from build123d import *

# Parameters (mm, degrees)
SKETCH_3_W          = 15
SKETCH_3_H          = 131.91272758
EXTRUDE_2_DEPTH     = 6.95
SKETCH_4_W          = 60
SKETCH_4_H          = 15
EXTRUDE_3_DEPTH     = 6.95
SKETCH_5_R          = 4.8
CUT_EXTRUDE_5_DEPTH = 7.95


with BuildPart() as part:
    # 草图3 → 凸台-拉伸2 (new body)
    with BuildSketch(Plane.XY):
        with Locations((-3.781807483, 0)):
            Rectangle(SKETCH_3_W, SKETCH_3_H)
    extrude(amount=EXTRUDE_2_DEPTH)

    # 草图4 → 凸台-拉伸3 (add)
    with BuildSketch(Plane.XY):
        with Locations((33.718192517, 58.45636379)):
            Rectangle(SKETCH_4_W, SKETCH_4_H)
    extrude(amount=EXTRUDE_3_DEPTH)

    # 草图5 → 切除-拉伸5 (cut, through all)
    with BuildSketch(Plane.XY):
        with Locations((-3.781807483, -54.073012812)):
            Circle(SKETCH_5_R)
    extrude(amount=CUT_EXTRUDE_5_DEPTH, mode=Mode.SUBTRACT)


solid = part.part
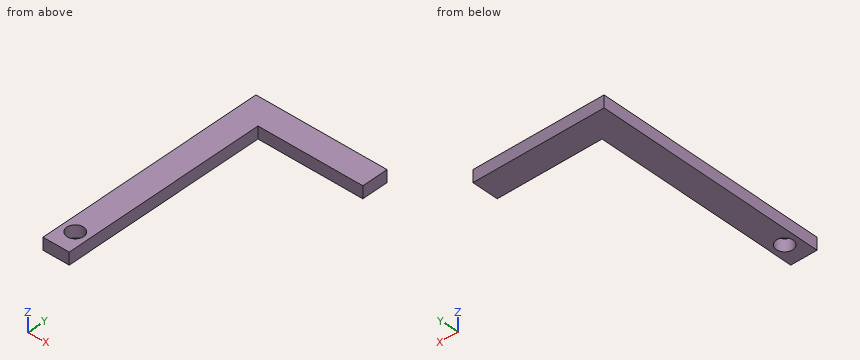
Design review of the part built by this model. Coordinates are the model's own, in mm. Give positions to 0.01 mm unless a question says otherwise; leave off trailing zeros. Loops run counter-clockwise (first coordinate to the right, second up) from the corner with the lowest first, then second, coordinate; pieces in that order, holes last. Notation, with made-up numbers: (6, 65) -> (17, 65) arc R21 ccw to (17, 98) -> close; hole circle Ø10 at (39, -28). An arc over 180 degrees is marked (long way). One line per question, with ' | ' between items. Start each with the question number.
(1) We need section C-C (z = 3.25). State the section outline as (x, y) points, and give its area (3 significant figures).
(2) For line 1 (X direction, y = 14, z = 4.25); line 2 (Y direction, x = 11.5, z = 3.25), list the stretches that pass through material, from the lowest coordinate up.
(3) We need section A-A (y = -51). State the section outline as (x, z) points.
(4) We need section B-B (x = -6). State the section outline as (y, z) points, and give its area (3 significant figures).
(5) We need section D-D (y = 26). State the section outline as (x, z) points.
(6) Insertion check: P1, Ø8.5, axis at x = -3.78, y = -54.07, coming from the +Z side; P2, Ø12, axis at x = 24, y = 46.5, coming from the -Z side; P3, Ø2, axis at y = -4, z = 4.5, coming from the +X side. Each pin has a flat end and moves straight along its axis. Give the tip position at first contact, or say it passes through.
The answers:
1) outline: (-11.28, -65.96) -> (3.72, -65.96) -> (3.72, 50.96) -> (63.72, 50.96) -> (63.72, 65.96) -> (-11.28, 65.96) -> close; hole circle Ø9.6 at (-3.78, -54.07) | area: 2,810 mm^2
2) line 1: x = -11.28 to 3.72 | line 2: y = 50.96 to 65.96
3) outline: (-11.28, 0) -> (-7.47, 0) -> (-7.47, 6.95) -> (-11.28, 6.95) -> close; (-0.09, 0) -> (3.72, 0) -> (3.72, 6.95) -> (-0.09, 6.95) -> close
4) outline: (-65.96, 0) -> (-58.33, 0) -> (-58.33, 6.95) -> (-65.96, 6.95) -> close; (-49.82, 0) -> (65.96, 0) -> (65.96, 6.95) -> (-49.82, 6.95) -> close | area: 858 mm^2
5) outline: (-11.28, 0) -> (3.72, 0) -> (3.72, 6.95) -> (-11.28, 6.95) -> close
6) P1: passes through | P2: stops at z = 0 | P3: stops at x = 3.72
